Source: CAD feature listing. Evaluate the final solid. Frame: model axes, mm. A direction names the side the tool comes from. Give positions to 0.01 mm unless a question says otherwise; leave off trailing zeros. Order: outer loops, then holes, each group sorted by start corner. A loop starts at its lowest first (then second) coordinate and runs counter-clockwise, first axis right, second up. Notation, with made-up numbers: (-8.75, 20.25) - (8.25, 20.25) arc R31 ccw to (8.25, 56.25) - close; hole circle Ø10 at (81.5, 65.5). An arc over 180 degrees is marked (long way). One line per item, written item: value. Start each with the question number.
from build123d import *

# Parameters (mm, degrees)
ESQUISSE1_R                                   = 9
BOSS_EXTRU_1_DEPTH                            = 4
ESQUISSE2_R                                   = 24
BOSS_EXTRU_2_DEPTH                            = 6
ESQUISSE7_R                                   = 7.5
BOSS_EXTRU_3_DEPTH                            = 50
TROU_POUR_TARAUDAGE_POUR_TROU_TARAUD_M4_D     = 3.3
TROU_POUR_TARAUDAGE_POUR_TROU_TARAUD_M4_DEPTH = 6
TROU_POUR_TARAUDAGE_POUR_TROU_TARAUD_M4_TIP   = 0.991420021
ENL_V_MAT_EXTRU_1_DEPTH                       = 3
TROU_POUR_TARAUDAGE_POUR_TROU_TARAUD_M6_D     = 5
TROU_POUR_TARAUDAGE_POUR_TROU_TARAUD_M6_DEPTH = 15
TROU_POUR_TARAUDAGE_POUR_TROU_TARAUD_M6_TIP   = 1.502151548


with BuildPart() as part:
    # Esquisse1 → Boss.-Extru.1 (new body)
    with BuildSketch(Plane.XY):
        Circle(ESQUISSE1_R)
    extrude(amount=BOSS_EXTRU_1_DEPTH)

    # Esquisse2 → Boss.-Extru.2 (add)
    with BuildSketch(Plane(origin=(0, 0, 0), x_dir=(-1, 0, 0), z_dir=(0, 0, -1))):
        Circle(ESQUISSE2_R)
    extrude(amount=BOSS_EXTRU_2_DEPTH)

    # Esquisse7 → Boss.-Extru.3 (add)
    with BuildSketch(Plane.XY.offset(4)):
        Circle(ESQUISSE7_R)
    extrude(amount=BOSS_EXTRU_3_DEPTH)

    # Trou pour taraudage pour trou taraudé M42
    with Locations(Plane(origin=(0, 0, -6), x_dir=(-1, 0, 0), z_dir=(0, 0, -1))):
        with Locations((-17, 9), (17, -9), (17, 9), (-17, -9)):
            Hole(TROU_POUR_TARAUDAGE_POUR_TROU_TARAUD_M4_D / 2, depth=TROU_POUR_TARAUDAGE_POUR_TROU_TARAUD_M4_DEPTH)
            with Locations((0, 0, -(TROU_POUR_TARAUDAGE_POUR_TROU_TARAUD_M4_DEPTH + TROU_POUR_TARAUDAGE_POUR_TROU_TARAUD_M4_TIP / 2))):  # 118° drill point
                Cone(0, TROU_POUR_TARAUDAGE_POUR_TROU_TARAUD_M4_D / 2, TROU_POUR_TARAUDAGE_POUR_TROU_TARAUD_M4_TIP, mode=Mode.SUBTRACT)

    # Esquisse10 → Enlèv. mat.-Extru.1 (cut)
    with BuildSketch(Plane.ZY.offset(7.5)):
        with BuildLine():
            Line((79, -2.5), (29, -2.5))
            ThreePointArc((29, -2.5), (26.5, 0), (29, 2.5))
            Line((29, 2.5), (79, 2.5))
            ThreePointArc((79, 2.5), (81.5, 0), (79, -2.5))
        make_face()
    extrude(amount=-ENL_V_MAT_EXTRU_1_DEPTH, mode=Mode.SUBTRACT)

    # Trou pour taraudage pour trou taraudé M61
    with Locations(Plane.XY.offset(54)):
        with Locations((0, 0)):
            Hole(TROU_POUR_TARAUDAGE_POUR_TROU_TARAUD_M6_D / 2, depth=TROU_POUR_TARAUDAGE_POUR_TROU_TARAUD_M6_DEPTH)
            with Locations((0, 0, -(TROU_POUR_TARAUDAGE_POUR_TROU_TARAUD_M6_DEPTH + TROU_POUR_TARAUDAGE_POUR_TROU_TARAUD_M6_TIP / 2))):  # 118° drill point
                Cone(0, TROU_POUR_TARAUDAGE_POUR_TROU_TARAUD_M6_D / 2, TROU_POUR_TARAUDAGE_POUR_TROU_TARAUD_M6_TIP, mode=Mode.SUBTRACT)


solid = part.part
1. Section B-B on z = 48.5. Return the cut outline in (x, y).
2. Contact query for flat-ended pins moving along their axis: pin 1 Ø10 at (y, z) = (0, 45) entering from -X; pin 2 Ø6 at (y, z) = (-4, 23) entering from +X; pin 3 Ø6 at (y, z) = (2, 24.5) entering from -X. Output: stop coordinate, or through.
3. Ray query, L1, parallel to Y at x = -17, z = -2; L2, parallel to X at y = 0, z = 47.25; L3, parallel to X at y = -9, z = -3.75. Return the intervals inside material, ascending.
4. Set-up query: faces 1 (the cylindrical face through (-15.476, 8.368, -2.958)), 2 (the cylindrical face through (-1.172, 8.923, 1.972)), 3 (the flat face through (-6, -2.5, 42)). Return all of +Z, -Z, +X, -X, +Y, -Y with unobstructed straight access to the full face (end or side cutting, diameter ignored); none if empty.
5. Section D-D on z = 11. Return the cut outline in (x, y).
6. Draft query along X for faces 4 (the cylindrical face through (18.574, -8.504, -2.958)), 5 (the flat face through (0, 0, -6)), 6 (the conical face through (-0.094, -0.424, 37.759)), 7 (the cylindrical face through (6.93, -2.87, 28.65)). Return one class per face: pulls with the +X half, pulls with the -X half, needs draft (parallel to the pull), parting line crosses it, or undercut.
7. Section A-A on x = -17. Return the cut outline in (y, z), then the cut area to 3 significant figures.
8. Section C-C on y = -16. Return the cut outline in (x, z).
Data:
1. outline: (-7.07, -2.5) arc R7.5 ccw (long way) to (-7.07, 2.5) - (-4.5, 2.5) - (-4.5, -2.5) - close; hole circle Ø5 at (0, 0)
2. pin 1: stops at x = -7.07
2. pin 2: stops at x = 7.43
2. pin 3: stops at x = -7.5
3. L1: y = -16.94 to -10.65, -7.35 to 7.35, 10.65 to 16.94
3. L2: x = -4.5 to -2.5, 2.5 to 7.5
3. L3: x = -22.25 to -18.65, -15.35 to 15.35, 18.65 to 22.25
4. face 1: +Z, -Z
4. face 2: +Z
4. face 3: +Z, -X
5. outline: circle Ø15 at (0, 0)
6. face 4: undercut
6. face 5: needs draft
6. face 6: undercut
6. face 7: parting line crosses it
7. outline: (-16.94, -6) - (-10.65, -6) - (-10.65, 0) - (-16.94, 0) - close; (-7.35, -6) - (7.35, -6) - (7.35, 0) - (-7.35, 0) - close; (10.65, -6) - (16.94, -6) - (16.94, 0) - (10.65, 0) - close
7. area: 164 mm2
8. outline: (-17.89, -6) - (17.89, -6) - (17.89, 0) - (-17.89, 0) - close
